Geometry check sheet. Reference: the model listing, model coordinates, mm. Round coordinates to 2 decimals unless told otherwise and drop trailing zeros. Order: outer loops, then holes, each group sorted by start corner. A loop starts at its lowest first (then second) coordinate and runs counter-clockwise, first axis right, second up. Notation, with made-up numbers: (-22.75, 67.25) -> (2.25, 67.25) arc R21 ccw to (2.25, 103.25) -> close; hole circle Ø2 at (5, 73.25). An arc over 180 degrees is marked (long way). Use a Markdown table: item, result. Add a question column.
Item 1: Gauge pin test, flat ends, axial feed: pin 1 Ø1 at (y, z) = (11.5, 1.5) entering from -X; pin 2 Ø1 at (x, y) = (29, 13) entering from -Z; pin 3 Ø1 at (x, z) = (23, 1) entering from +Y; pin 4 Ø1 at (y, z) = (13.5, 1) entering from +X. Record the tip position at first contact, or that the pin passes through.
Item 2: Sectioned sample at A-A, the plane y = 15. Record the cut outline in (x, z).
Item 3: Sectioned sample at D-D, the plane x = 42.5. Record the cut outline in (y, z).
Item 4: Sectioned sample at C-C, the plane z = 0.65. Record the cut outline in (x, y), and give its area (3 significant figures).
Item 5: Sectioned sample at B-B, the plane y = -15. Record the cut outline in (x, z), and give its area (3 significant figures).
Item 6: Material ranges on probe 1 along X at (y, z) = (14, 1.9); probe 2 along Y at (x, z) = (7, 1.15); probe 3 along X at (y, z) = (-15, 1.05), recorded low to high. Write a range as [from, to].
Autodesk Inventor part; units mm, degrees
ref_plane "YZ Plane" through (0, 0, 0) normal (1, 0, 0) x (0, 1, 0)
ref_plane "XZ Plane" through (0, 0, 0) normal (0, 1, 0) x (-1, 0, 0)
ref_plane "XY Plane" through (0, 0, 0) normal (0, 0, 1) x (1, 0, 0)
ref_plane "Arbeitsebene1" through (0, 0, 0) normal (0, 0, 1) x (1, 0, 0)
sketch "Skizze1" plane through (0, 0, 0) normal (0, 0, 1) x (1, 0, 0)
  line L0 (8.0712, 15) -> (38.0712, 15)
  line L1 (38.0712, 15) -> (38.0712, -15)
  line L2 (38.0712, -15) -> (8.0712, -15)
  line L3 (8.0712, -15) -> (8.0712, 15)
  line L4 (38.0712, 19) -> (8.0712, 19)
  line L5 (4.0712, 15) -> (4.0712, -15)
  line L6 (8.0712, -19) -> (38.0712, -19)
  line L7 (42.0712, -15) -> (42.0712, 15)
  arc A0 (8.0712, 19) -> (4.0712, 15) centre (8.0712, 15) ccw
  arc A1 (42.0712, 15) -> (38.0712, 19) centre (38.0712, 15) ccw
  arc A2 (38.0712, -19) -> (42.0712, -15) centre (38.0712, -15) ccw
  arc A3 (4.0712, -15) -> (8.0712, -19) centre (8.0712, -15) ccw
  line L8 (29.9712, -18.3074) -> (29.9712, -24.4)
  circle A4 centre (38.0712, -15) radius 1.4
  circle A5 centre (38.0712, 15) radius 1.4
  line L9 (39.5712, -24.4) -> (29.9712, -24.4)
  line L10 (39.5712, -21.1181) -> (39.5712, -24.4)
  line L11 (44.1893, -16.5) -> (39.5712, -21.1181)
  line L12 (47.4712, -16.5) -> (44.1893, -16.5)
  line L13 (47.4712, 16.5) -> (47.4712, -16.5)
  line L14 (44.1893, 16.5) -> (47.4712, 16.5)
  line L15 (39.5712, 21.1181) -> (44.1893, 16.5)
  line L16 (39.5712, 24.4) -> (39.5712, 21.1181)
  line L17 (31.5712, 24.4) -> (39.5712, 24.4)
  line L18 (31.5712, 4.0068) -> (31.5712, 24.4)
  arc A6 (32.7786, 1.7) -> (31.5712, 4.0068) centre (29.9712, 1.7) ccw
  line L19 (32.7786, 1.7) -> (32.7786, -15.5)
  arc A7 (29.9712, -18.3074) -> (32.7786, -15.5) centre (29.9712, -15.5) ccw
  arc A8 (16.5712, 25.149) -> (3.3138, -16.9) centre (23.0897, -0.0206) ccw
  circle A9 centre (23.0897, -0.0206) radius 26
  point P0 (0, 0)
  point P1 (36.5793, -24.4)
  point P2 (31.5712, 11.3758)
  point P3 (3.3138, -16.9)
  dimension "d0" = 4
  dimension "d1" = 4
extrude "Extrusion1" add sketch "Skizze1" along normal blind 2 contours L3 L2 L19 A7 L8 L6 A3 L5 A0 L4 L18 L0 | L0 L18 A6 L19 L2 L3 | L18 L4 A1 L7 A2 L6 L8 A7 L19 L2 A4 L1 A5 L0 | L0 A5 L1 A4 L2 L19 A6 L18 | A5 L1 L0 | L0 L1 A5 | L18 L17 A9 L13 L9 L8 L6 A2 L7 A1 L4 | L4 A0 L5 A3 L6 L8 L9 A9 A8 L17 L18 | A4 L1 L2 | L2 L1 A4 | A9 L13
ref_plane "Arbeitsebene2" through (0, 0, 0) normal (0, 0, 1) x (1, 0, 0)
sketch "Skizze2" plane through (0, 0, 2) normal (0, 0, 1) x (1, 0, 0)
  arc A0 (8.0712, 19) -> (4.0712, 15) centre (8.0712, 15) ccw
  line L0 (4.0712, 15) -> (4.0712, -15)
  arc A1 (4.0712, -15) -> (8.0712, -19) centre (8.0712, -15) ccw
  line L1 (8.0712, -19) -> (38.0712, -19)
  arc A2 (38.0712, -19) -> (42.0712, -15) centre (38.0712, -15) ccw
  line L2 (42.0712, -15) -> (42.0712, 15)
  arc A3 (42.0712, 15) -> (38.0712, 19) centre (38.0712, 15) ccw
  line L3 (38.0712, 19) -> (8.0712, 19)
  circle A4 centre (8.0712, 15) radius 1.4
  circle A5 centre (38.0712, 15) radius 1.4
  circle A6 centre (38.0712, -15) radius 1.4
  circle A7 centre (8.0712, -15) radius 1.4
  point P0 (0, 0)
hole "Bohrung1" at (8.0712, 15, 2) at (8.0712, -15, 2) at (38.0712, -15, 2) at (38.0712, 15, 2) direction (0, 0, -1) diameter 3.2 end through all
sketch "Skizze3" plane through (0, 0, 2) normal (0, 0, 1) x (1, 0, 0)
  circle A0 centre (23.0919, -0.0207) radius 4.25
  arc A1 (30.2483, 24.4) -> (29.5712, 22.9) centre (31.5712, 22.9) ccw
  line L0 (39.5712, 24.4) -> (30.2483, 24.4)
  line L1 (39.5712, 21.1181) -> (39.5712, 24.4)
  line L2 (44.1893, 16.5) -> (39.5712, 21.1181)
  line L3 (47.4712, 16.5) -> (44.1893, 16.5)
  line L4 (47.4712, -16.5) -> (47.4712, 16.5)
  line L5 (44.1893, -16.5) -> (47.4712, -16.5)
  line L6 (39.5712, -21.1181) -> (44.1893, -16.5)
  line L7 (39.5712, -24.4) -> (39.5712, -21.1181)
  line L8 (6.6126, -24.4) -> (39.5712, -24.4)
  line L9 (6.6126, -21.1595) -> (6.6126, -24.4)
  line L10 (1.9531, -16.5) -> (6.6126, -21.1595)
  line L11 (-1.3288, -16.5) -> (1.9531, -16.5)
  line L12 (-1.3288, 16.5) -> (-1.3288, -16.5)
  line L13 (1.9531, 16.5) -> (-1.3288, 16.5)
  line L14 (6.5712, 21.1181) -> (1.9531, 16.5)
  line L15 (6.5712, 24.4) -> (6.5712, 21.1181)
  line L16 (15.894, 24.4) -> (6.5712, 24.4)
  arc A2 (16.5712, 22.9) -> (15.894, 24.4) centre (14.5712, 22.9) ccw
  line L17 (16.5712, 22.9) -> (16.5712, 6.5074)
  arc A3 (16.5712, 6.5074) -> (18.5712, 4.5074) centre (18.5712, 6.5074) ccw
  line L18 (18.5712, 4.5074) -> (27.5712, 4.5074)
  arc A4 (27.5712, 4.5074) -> (29.5712, 6.5074) centre (27.5712, 6.5074) ccw
  line L19 (29.5712, 6.5074) -> (29.5712, 22.9)
  circle A5 centre (38.0712, 15) radius 1.4
  circle A6 centre (8.0712, -15) radius 1.4
  circle A7 centre (38.0712, -15) radius 1.4
  circle A8 centre (8.0712, 15) radius 1.4
  line L20 (15.894, 24.4) -> (30.2483, 24.4)
  line L21 (6.5712, 24.4) -> (39.5712, 24.4)
  line L22 (39.5712, 24.4) -> (39.5712, 27.6612)
  line L23 (39.5712, 27.6612) -> (6.5712, 27.6612)
  line L24 (6.5712, 27.6612) -> (6.5712, 24.4)
  point P0 (0, 0)
extrude "Extrusion2" cut sketch "Skizze3" against normal blind 10 contours L20 L16 L24 L23 L22 L0 | A1 L19 A4 L18 A3 L17 A2 L20
fillet "Rundung1" [suppressed]
properties part number "20_Cube_Insert_SEEED_Xiao_Sense_Camera_backplate"
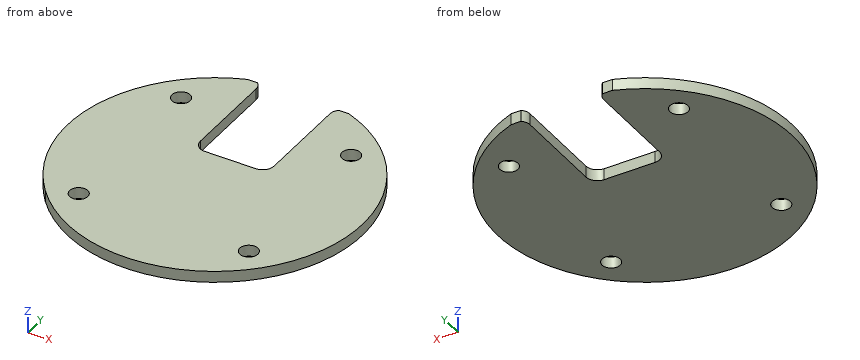
Found:
| question | item | result |
|---|---|---|
| 1 | pin 1 | stops at x = -0.46 |
| 1 | pin 2 | passes through |
| 1 | pin 3 | stops at y = 4.51 |
| 1 | pin 4 | stops at x = 45.59 |
| 2 | outline | (1.87, 0) -> (6.47, 0) -> (6.47, 2) -> (1.87, 2) -> close; (9.67, 0) -> (16.57, 0) -> (16.57, 2) -> (9.67, 2) -> close; (29.57, 0) -> (36.47, 0) -> (36.47, 2) -> (29.57, 2) -> close; (39.67, 0) -> (44.31, 0) -> (44.31, 2) -> (39.67, 2) -> close |
| 3 | outline | (-17.32, 0) -> (17.28, 0) -> (17.28, 2) -> (-17.32, 2) -> close |
| 4 | outline | (3.31, -16.9) arc R26 ccw (long way) to (32.01, 24.4) -> (30.25, 24.4) arc R2 ccw to (29.57, 22.9) -> (29.57, 6.51) arc R2 cw to (27.57, 4.51) -> (18.57, 4.51) arc R2 cw to (16.57, 6.51) -> (16.57, 22.9) arc R2 ccw to (15.89, 24.4) -> (14.17, 24.4) arc R26 ccw to start; hole circle Ø3.2 at (8.07, -15); hole circle Ø3.2 at (8.07, 15); hole circle Ø3.2 at (38.07, -15); hole circle Ø3.2 at (38.07, 15) |
| 4 | area | 1,820 mm2 |
| 5 | outline | (1.84, 0) -> (6.47, 0) -> (6.47, 2) -> (1.84, 2) -> close; (9.67, 0) -> (36.47, 0) -> (36.47, 2) -> (9.67, 2) -> close; (39.67, 0) -> (44.34, 0) -> (44.34, 2) -> (39.67, 2) -> close |
| 5 | area | 72.2 mm2 |
| 6 | probe 1 | x = [1.19, 6.82], [9.32, 16.57], [29.57, 36.82], [39.32, 44.99] |
| 6 | probe 2 | y = [-20.44, -16.19], [-13.81, 13.81], [16.19, 20.4] |
| 6 | probe 3 | x = [1.84, 6.47], [9.67, 36.47], [39.67, 44.34] |
